Check sheet for the drawn part. Datum: minimum x, y, z corner. Units: mm. A direction names the side the tool comes from. Coordinates: 2 decimals unless noted, no trailing zeros. Write each loop counter-clockwise with the first axis right and the second up, starting at its lowest first coordinate (ties: lowest second). Pieces come first, ordered by that corner, then holes. Notation, with made-up numbers: M 62,70.5 L 98,70.5 A29 cw 98,103.5 Z; hole C 56.5,84.25 d9. An arc over 180 degrees is marked long. Answer as a JSON object with one key per item and string values. Group by question number.
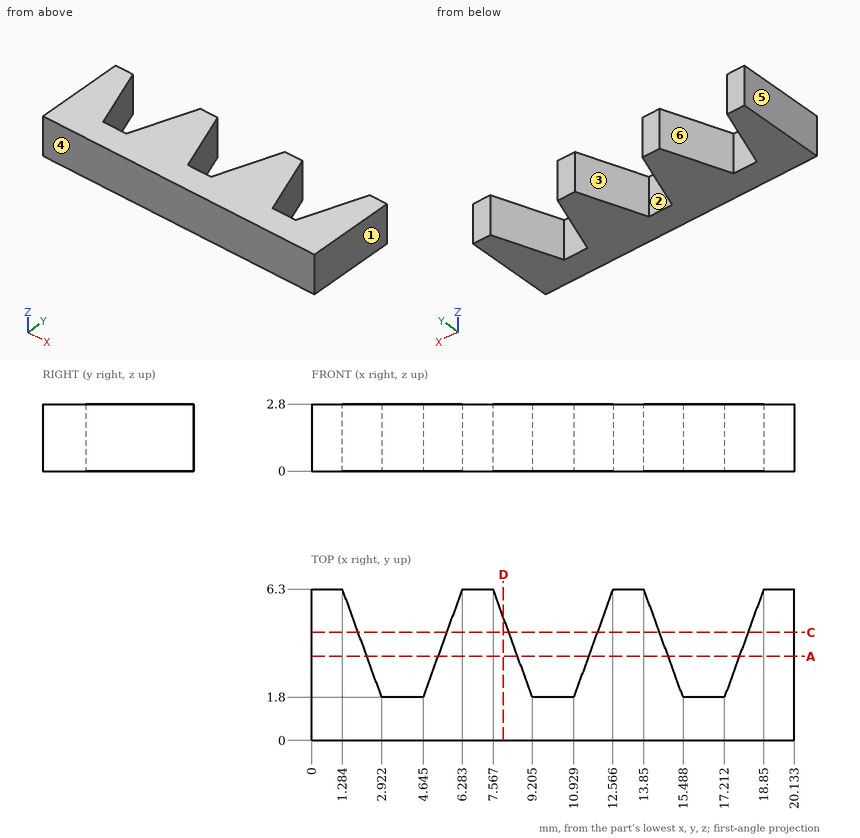
1) Set-up check for the marked faces 5 and 6: record each of +Z, -Z, +X, -X, +Y, -Y from which the full face is reachable in a straight line by a thin tool's end or side.
2) Go/stop test with a flat-tipped pin: pin 1 Ø0.5 at (x, z) = (10, 2) entering from +Y. Record where the tip stops, or that it passes through.
3) Section check A-A (y = 3.5). Record the cut outline in (x, z) (1 decimal).
4) Section check D-D (x = 8). Record the cut outline in (y, z).
5) Draft check along X on the marked faces 1, 2, 3 and 4. Enter one of: +X half, -X half, draft (parallel to the pull), parting line (faces both ways), or undercut.
6) Section check C-C (y = 4.5). Record the cut outline in (x, z) (1 decimal).
7) Material ranges on probe 1 along X at (y, z) = (4.5, 2.05) (1 decimal); probe 2 along X at (y, z) = (2.25, 0.6) (1 decimal); probe 3 along Y at (x, z) = (9.5, 0.9), recorded low to high. Write a range as [from, to].
Entries:
{
 "1": {"face 5": "+Z, -Z, -X, +Y, -Y", "face 6": "+Z, -Z, +Y"},
 "2": {"pin 1": "y = 1.8"},
 "3": {"outline": "M 0,0 L 2.3,0 L 2.3,2.8 L 0,2.8 Z; M 5.3,0 L 8.6,0 L 8.6,2.8 L 5.3,2.8 Z; M 11.5,0 L 14.9,0 L 14.9,2.8 L 11.5,2.8 Z; M 17.8,0 L 20.1,0 L 20.1,2.8 L 17.8,2.8 Z"},
 "4": {"outline": "M 0,0 L 5.11,0 L 5.11,2.8 L 0,2.8 Z"},
 "5": {"face 1": "+X half", "face 2": "undercut", "face 3": "undercut", "face 4": "draft"},
 "6": {"outline": "M 0,0 L 1.9,0 L 1.9,2.8 L 0,2.8 Z; M 5.6,0 L 8.2,0 L 8.2,2.8 L 5.6,2.8 Z; M 11.9,0 L 14.5,0 L 14.5,2.8 L 11.9,2.8 Z; M 18.2,0 L 20.1,0 L 20.1,2.8 L 18.2,2.8 Z"},
 "7": {"probe 1": "[0, 1.9], [5.6, 8.2], [11.9, 14.5], [18.2, 20.1]", "probe 2": "[0, 2.8], [4.8, 9], [11.1, 15.3], [17.4, 20.1]", "probe 3": "[0, 1.8]"}
}
